```python
from build123d import *

# Parameters (mm, degrees)
F1_DEPTH = 15


# Not quite as in the source:
# - a feature names something its author has since deleted; it is built from what else it names


with BuildPart() as f1:
    # F0 (on Front) → F1 (new body)
    with BuildSketch(Plane.XZ):
        with BuildLine():
            Line((45.2788062093, 66.612446636), (-16.9345241785, 66.612446636))
            ThreePointArc((-16.9345241785, 66.612446636), (-20.4700580844, 65.1479805419), (-21.9345241785, 61.612446636))
            Line((-21.9345241785, 61.612446636), (-21.9345241785, 21.612446636))
            ThreePointArc((-21.9345241785, 21.612446636), (-20.4700580844, 18.07691273), (-16.9345241785, 16.612446636))
            Line((-16.9345241785, 16.612446636), (-12.2681620345, 16.612446636))
            ThreePointArc((-12.2681620345, 16.612446636), (-4.7681620345, 9.112446636), (2.7318379655, 16.612446636))
            Line((2.7318379655, 16.612446636), (51.954228729, 16.612446636))
            ThreePointArc((51.954228729, 16.612446636), (59.454228729, 9.112446636), (66.954228729, 16.612446636))
            Line((66.954228729, 16.612446636), (69.8528067806, 16.612446636))
            ThreePointArc((69.8528067806, 16.612446636), (73.0579467169, 17.774859114), (74.7728087909, 20.7216154405))
            ThreePointArc((74.7728087909, 20.7216154405), (69.0623483383, 49.4748090163), (45.2788062093, 66.612446636))
        make_face()
        with BuildLine():
            ThreePointArc((-14.2601495609, 59.612446636), (-13.3814699044, 61.7337669795), (-11.2601495609, 62.612446636))
            Line((-11.2601495609, 62.612446636), (2.1277400926, 62.612446636))
            ThreePointArc((2.1277400926, 62.612446636), (4.2490604361, 61.7337669795), (5.1277400926, 59.612446636))
            Line((5.1277400926, 59.612446636), (5.1277400926, 43.612446636))
            ThreePointArc((5.1277400926, 43.612446636), (4.2490604361, 41.4911262924), (2.1277400926, 40.612446636))
            Line((2.1277400926, 40.612446636), (-11.2601495609, 40.612446636))
            ThreePointArc((-11.2601495609, 40.612446636), (-13.3814699044, 41.4911262924), (-14.2601495609, 43.612446636))
            Line((-14.2601495609, 43.612446636), (-14.2601495609, 59.612446636))
        make_face(mode=Mode.SUBTRACT)
        with BuildLine():
            ThreePointArc((11.388416402, 59.612446636), (12.2670960585, 61.7337669795), (14.388416402, 62.612446636))
            Line((14.388416402, 62.612446636), (34.4408885837, 62.612446636))
            ThreePointArc((34.4408885837, 62.612446636), (36.5622089272, 61.7337669795), (37.4408885837, 59.612446636))
            Line((37.4408885837, 59.612446636), (37.4408885837, 43.612446636))
            ThreePointArc((37.4408885837, 43.612446636), (36.5622089272, 41.4911262924), (34.4408885837, 40.612446636))
            Line((34.4408885837, 40.612446636), (14.388416402, 40.612446636))
            ThreePointArc((14.388416402, 40.612446636), (12.2670960585, 41.4911262924), (11.388416402, 43.612446636))
            Line((11.388416402, 43.612446636), (11.388416402, 59.612446636))
        make_face(mode=Mode.SUBTRACT)
        with BuildLine():
            ThreePointArc((61.6208599434, 43.4263003167), (60.6810944136, 41.4263040334), (58.626640588, 40.612446636))
            Line((58.626640588, 40.612446636), (46.5931359261, 40.612446636))
            ThreePointArc((46.5931359261, 40.612446636), (44.4718155826, 41.4911262924), (43.5931359261, 43.612446636))
            Line((43.5931359261, 43.612446636), (43.5931359261, 59.3101777172))
            ThreePointArc((43.5931359261, 59.3101777172), (44.6949543188, 61.6333020328), (47.1910736498, 62.2499856155))
            ThreePointArc((47.1910736498, 62.2499856155), (57.9277499616, 55.5378575882), (61.6208599434, 43.4263003167))
        make_face(mode=Mode.SUBTRACT)
    extrude(amount=F1_DEPTH)


solid = f1.part
```
CAD build for the part. Positions are in the model's coordinates, mm. A direction names the side the tool comes from. Round coordinates to 2 decimals unless told otherwise and drop trailing zeros. Loops run counter-clockwise (first coordinate to the right, second up) from the corner with the lowest first, then second, coordinate; pieces in that order, holes last. Notation, with made-up numbers: M 54.5,-31.75 L 76.5,-31.75 A30 cw 76.5,-1.75 Z; hole C -24,-14 d11. An arc over 180 degrees is marked long. Return JSON: item names as keys, results as strings. Group by question number.
(1) Tool access for faces 1 (the flat face through (15, -7, 66.612)), 2 (the flat face through (25, -7, 40.612)), 3 (the flat face through (27, -7, 16.612)): list every direction of +Z, -Z, +X, -X, +Y, -Y with a clear straight run to the whole face (end or side of a thin tool).
(2) Saw through at C-C, the plane x = 55. List the corners of the cut face in (y, z).
(3) Saw through at B-B, the plane y = -3.25. Give the number of separate pieces and of enclosed holes in the cut face, and give its area (3 significant figures).
(4) Wall check: probe 1 along Z at (x, y) = (23, -0.75); probe 2 along X at (y, z) = (-11, 44); probe 3 along X at (y, z) = (-14, 51.5). Give the ranges that are in metal, low to high. Write a range as [from, to].
(5) Drop flat-ended pins along their axis: P1, Ø4.5, axis at y = -4.5, z = 51.5, coming from the +X side; P2, Ø1.4, axis at x = 68.5, y = -11, coming from the -Z side; P3, Ø5, axis at x = -10.5, y = -7, coming from the -Z side. Give the stop position or say it passes through.
(6) Saw through at A-A, the plane x = 15.5. List the corners of the cut face in (y, z).
(7) Mould opens along X. For faces 4 (the flat face through (68, -7, 16.612)), 5 (the flat face through (-5, -7, 62.612)), 6 (the cylindrical face through (4.27, -7.4, 41.51)), 7 (the cylindrical face through (69.3, -7.4, 49.1)) say: +X half, -X half, draft (parallel to the pull), parting line (faces both ways), or undercut.
Answer list:
{
 "1": {"face 1": "+Z, +X, -X, +Y, -Y", "face 2": "+Y, -Y", "face 3": "-Z, +Y, -Y"},
 "2": {"outline": "M -15,10.58 L 0,10.58 L 0,40.61 L -15,40.61 Z; M -15,58.55 L 0,58.55 L 0,62.72 L -15,62.72 Z"},
 "3": {"separate pieces": "1", "enclosed holes": "3", "area": "3,420 mm2"},
 "4": {"probe 1": "[16.61, 40.61], [62.61, 66.61]", "probe 2": "[-21.93, -14.26], [5.13, 11.39], [37.44, 43.59], [61.65, 72.01]", "probe 3": "[-21.93, -14.26], [5.13, 11.39], [37.44, 43.59], [60.26, 67.67]"},
 "5": {"P1": "x = 69.21", "P2": "z = 16.61", "P3": "z = 9.84"},
 "6": {"outline": "M -15,16.61 L 0,16.61 L 0,40.61 L -15,40.61 Z; M -15,62.61 L 0,62.61 L 0,66.61 L -15,66.61 Z"},
 "7": {"face 4": "draft", "face 5": "undercut", "face 6": "undercut", "face 7": "+X half"}
}
